```python
from build123d import *

# Parameters (mm, degrees)
F1_DEPTH = 1.016
F2_SIZE2 = 2
F2_SIZE  = 1
F3_SIZE2 = 1
F3_SIZE  = 2


with BuildPart() as f1:
    # F0 (on Top) → F1 (new body, symmetric)
    with BuildSketch(Plane.XY):
        with BuildLine():
            Line((51.551948, 26.457513), (34.29, 24.0665))
            Line((34.29, 24.0665), (-22.987, 24.0665))
            ThreePointArc((-22.987, 24.0665), (-25.232064, 23.136564), (-26.162, 20.8915))
            Line((-26.162, 20.8915), (-26.162, 19.7485))
            ThreePointArc((-26.162, 19.7485), (-25.232064, 17.503436), (-22.987, 16.5735))
            Line((-22.987, 16.5735), (-8.73125, 16.5735))
            ThreePointArc((-8.73125, 16.5735), (-6.35, 18.95475), (-3.96875, 16.5735))
            Line((-3.96875, 16.5735), (34.29, 16.5735))
            Line((34.29, 16.5735), (51.551948, 14.182487))
            ThreePointArc((51.551948, 14.182487), (52.648713, 13.589108), (53.086, 12.421302))
            Line((53.086, 12.421302), (53.086, 11.43))
            Line((53.086, 11.43), (59.436, 11.43))
            Line((59.436, 11.43), (108.966, 11.43))
            ThreePointArc((108.966, 11.43), (131.577707, 15.010048), (151.977583, 25.4))
            Line((151.977583, 25.4), (108.966, 29.21))
            Line((108.966, 29.21), (59.436, 29.21))
            Line((59.436, 29.21), (53.086, 29.21))
            Line((53.086, 29.21), (53.086, 28.218698))
            ThreePointArc((53.086, 28.218698), (52.648713, 27.050892), (51.551948, 26.457513))
        make_face()
    extrude(amount=F1_DEPTH, both=True)

    # F2
    f2_edges = [f1.edges().sort_by_distance(p)[0] for p in [
        (81.026, 11.43, 1.016),
    ]]
    chamfer(f2_edges, length=F2_SIZE, length2=F2_SIZE2)

    # F3
    f3_edges = [f1.edges().sort_by_distance(p)[0] for p in [
        (81.026, 11.43, -1.016),
    ]]
    chamfer(f3_edges, length=F3_SIZE, length2=F3_SIZE2)


solid = f1.part
```
Can you work these out from the model? Positions are in its coordinate system, mm. Round coordinates to 2 decimals unless told otherwise and drop trailing zeros. Loops run counter-clockwise (first coordinate to the right, second up) from the corner with the lowest first, then second, coordinate; pieces in that order, holes last. Notation, with made-up numbers: M -38.5,-23.5 L -5.5,-23.5 A29 ccw -5.5,5.5 Z; hole C 89,-24.75 d9. An arc over 180 degrees is marked long. Write item = value, one per line. Start each with the question number.
(1) Suppose I cut it at B-B on x = -6.35. Write out the boundary of the cut face in (y, z), plus the area to 3 significant figures.
(2) Suppose I cut it at C-C on x = 39. Write out the boundary of the cut face in (y, z), plus the area to 3 significant figures.
(3) I'm going to push flat-ended pins straight in: P1, Ø1.1, axis at y = 12, z = 0, coming from the -X side; P2, Ø0.6, axis at x = -14.5, z = 0.5, coming from the -Y side. Where does each tip first touch, or does it pass through?
(4) I need wall thicknesses on line 1 along Y through (x, z) = (27.5, 0); line 2 along Y through (x, z) = (34.5, 0.85). Which ranges of each line are inside material? Lowest first, please.
Answer block:
q1.outline = M 18.95,-1.02 L 24.07,-1.02 L 24.07,1.02 L 18.95,1.02 Z
q1.area = 10.4 mm²
q2.outline = M 15.92,-1.02 L 24.72,-1.02 L 24.72,1.02 L 15.92,1.02 Z
q2.area = 17.9 mm²
q3.P1 = 53.08
q3.P2 = 16.57
q4.line_1 = 16.57 to 24.07
q4.line_2 = 16.54 to 24.1
